Geometry check sheet. Reference: drawing and pictorial views, mm from the part's lowest x, y, z. A direction names the side the tool comes from. Round coordinates to 2 decimals unless told otherwise and drop trailing zeros. Loops run counter-clockwise (first coordinate to the right, second up) from the corner with the lowest first, then second, coordinate; pieces in that order, holes last. Notation, with made-up numbers: (-40, -28) - (-16, -28) arc R15 cw to (-16, -24) - close; hole circle Ø10 at (74.5, 45). An arc over 180 degrees is marked (long way). Return JSON: item names as keys, results as strings.
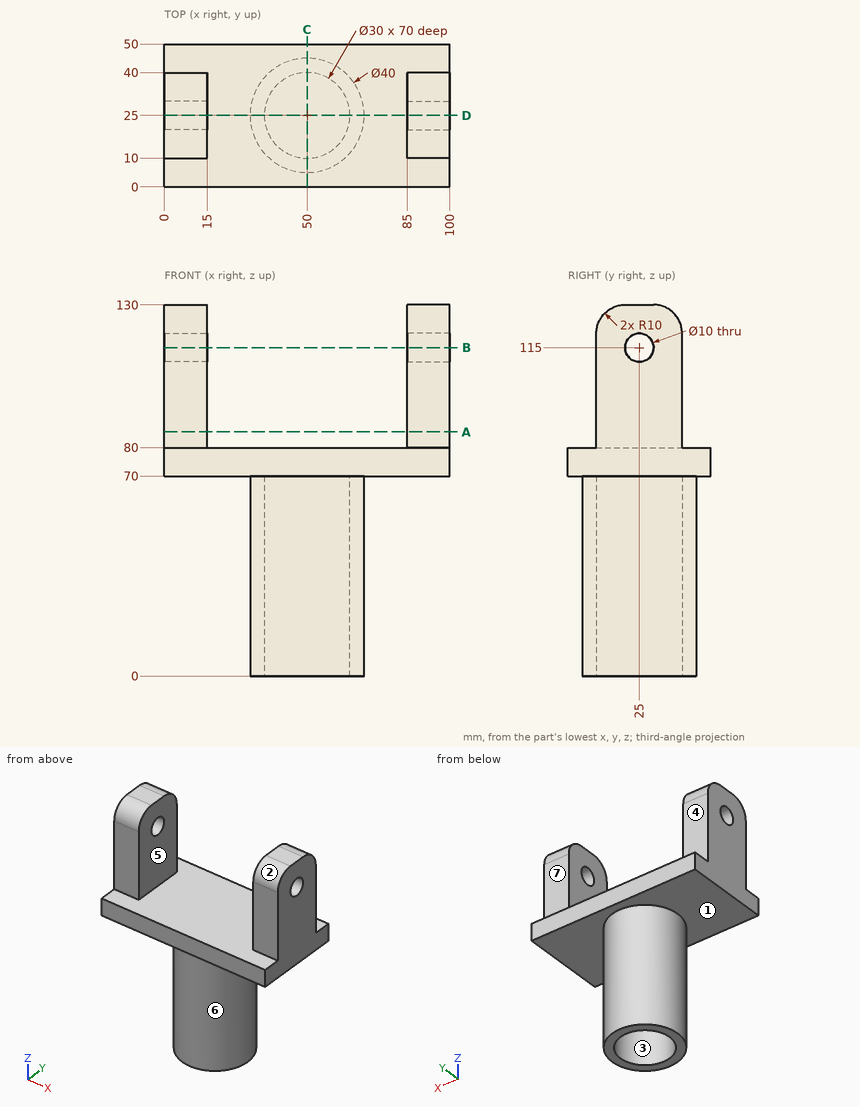
Q1. Scan lines: probe 1 along X at (y, z) = (34, 92.5); probe 2 along Y at (x, z) = (50, 19); probe 3 along Z at (x, y) = (90, 25). Record each from-to range of solid material in increasing order. Write a range as [from, to].
Answer key:
{"probe 1": "x = [0, 15], [85, 100]", "probe 2": "y = [5, 10], [40, 45]", "probe 3": "z = [70, 110], [120, 130]"}
Q2. Depth check by flat-ended pin: P1, Ø4.5, axis at x = 94, z = 105.5, coming from the +Y side; P2, Ø24, axis at x = 50, y = 25, coming from the +Z side; P3, Ø9, axis at y = 25, z = 115, coming from the +X side; P4, Ø10, axis at x = 29, z = 42, coming from the -Y side. Enter the tip coordinate at first touch or a pass-through.
Answer key:
{"P1": "stops at y = 40", "P2": "stops at z = 80", "P3": "passes through", "P4": "stops at y = 13"}
Q3. Sectioned sample at C-C (x = 50). Enter the section's corners in (y, z).
Answer key:
{"outline": "(0, 70) - (5, 70) - (5, 0) - (10, 0) - (10, 70) - (40, 70) - (40, 0) - (45, 0) - (45, 70) - (50, 70) - (50, 80) - (0, 80) - close"}
Q4. Sectioned sample at D-D (y = 25). Enter the section's corners in (x, z), plus the area to 3 significant figures.
Answer key:
{"outline": "(0, 70) - (30, 70) - (30, 0) - (35, 0) - (35, 70) - (65, 70) - (65, 0) - (70, 0) - (70, 70) - (100, 70) - (100, 110) - (85, 110) - (85, 80) - (15, 80) - (15, 110) - (0, 110) - close; (0, 120) - (15, 120) - (15, 130) - (0, 130) - close; (85, 120) - (100, 120) - (100, 130) - (85, 130) - close", "area": "2,900 mm²"}
Q5. Tool access check on the marked faces 5, 6 and 7. Record the directions out of +Z, -Z, +X, -X, +Y, -Y that give a thin tool (end or side, any length) a straight path to the whole face; none if there is none.
Answer key:
{"face 5": "+Z, +Y, -Y", "face 6": "-Z", "face 7": "+Z, +X, -X, +Y"}
Q6. Draft check along Y on the marked faces 1, 2, 3 and 4. Enter one of: released by +Y, released by -Y, zero draft, split by the parting line, or undercut.
Answer key:
{"face 1": "zero draft", "face 2": "released by -Y", "face 3": "undercut", "face 4": "released by +Y"}
Q7. Sectioned sample at A-A (z = 85.5). Enter the section's corners in (x, y), plus the area to 3 significant figures.
Answer key:
{"outline": "(0, 10) - (15, 10) - (15, 40) - (0, 40) - close; (85, 10) - (100, 10) - (100, 40) - (85, 40) - close", "area": "900 mm²"}
Q8. Sectioned sample at B-B (z = 115). Enter the section's corners in (x, y), plus the area to 3 significant figures.
Answer key:
{"outline": "(0, 10) - (15, 10) - (15, 20) - (0, 20) - close; (0, 30) - (15, 30) - (15, 40) - (0, 40) - close; (85, 10) - (100, 10) - (100, 20) - (85, 20) - close; (85, 30) - (100, 30) - (100, 40) - (85, 40) - close", "area": "600 mm²"}
